Could you check a few things on this model? Use its own coordinates, in mm. Coordinates: 2 decimals unless noted, no trailing zeros. Loops run counter-clockwise (first coordinate to the right, second up) from the corner with the lowest first, then second, coordinate; pieces in that order, holes last.
from build123d import *

# Parameters (mm, degrees)
BOSS_EXTRUDE1_DEPTH = 3.175
SKETCH4_R           = 6.35
BOSS_EXTRUDE2_DEPTH = 3.175


with BuildPart() as part:
    # Sketch3 → Boss-Extrude1 (new body)
    with BuildSketch(Plane(origin=(0, 42.21734, 0), x_dir=(1, 0, 0), z_dir=(0, 1, 0))):
        with BuildLine():
            Line((35.908808919, 4.798625676), (-36.070576217, 67.18075946))
            ThreePointArc((-36.070576217, 67.18075946), (-45.028010811, 66.540942703), (-44.388194055, 57.583508109))
            Line((-44.388194055, 57.583508109), (27.591191081, -4.798625676))
            ThreePointArc((27.591191081, -4.798625676), (36.548625676, -4.158808919), (35.908808919, 4.798625676))
        make_face()
    extrude(amount=-BOSS_EXTRUDE1_DEPTH)

    # Sketch4 → Boss-Extrude2 (add)
    with BuildSketch(Plane.XZ.offset(-39.04234)):
        with Locations((-40.229385136, -62.382133784)):
            Circle(SKETCH4_R)
    extrude(amount=BOSS_EXTRUDE2_DEPTH)


solid = part.part
1) Will these pins go through, and if not, where does the flat tip stop? pin 1 (1.5 mm diameter, centred on x = -3, y = 41, fed in from +Z); pin 2 (22 mm diameter, centred on x = -15.5, z = -41, fed in from -Y); pin 3 (1.5 mm diameter, centred on x = -11, y = 37.5, fed in from +Z).
2) Imagine slicing it at B-B on x = -39.5. List the corners of the cut face in (y, z) for me, plus the area to 3 significant figures.
3) Imagine slicing it at C-C on z = 0. List the corners of the cut face in (x, y) for me, plus the area to 3 significant figures.
4) If I drill on L1, parallel to Y at x = 21.5, z = -4.5; L2, parallel to X at y = 38, z = -62; L3, parallel to X at y = 40.5, z = -14.5, over which ranges is the centre line in solid material (lowest first)?
5) Imagine slicing it at A-A on y = 41. List the corners of the cut face in (x, z) for me.
Solved:
1. pin 1: stops at z = -21.06
1. pin 2: stops at y = 39.04
1. pin 3: passes through
2. outline: (35.87, -68.69) - (42.22, -68.69) - (42.22, -53.35) - (39.04, -53.35) - (39.04, -56.07) - (35.87, -56.07) - close
2. area: 88.8 mm2
3. outline: (22.05, 39.04) - (38.1, 39.04) - (38.1, 42.22) - (22.05, 42.22) - close
3. area: 50.9 mm2
4. L1: y = 39.04 to 42.22
4. L2: x = -46.57 to -33.89
4. L3: x = 5.32 to 24.71
5. outline: (-44.39, -57.58) arc R6.35 ccw to (-36.07, -67.18) - (35.91, -4.8) arc R6.35 ccw to (27.59, 4.8) - close
